from build123d import *

# Parameters (mm, degrees)
F0_R     = 88.9
F1_DEPTH = 50.8
F2_SIZE  = 25.4
F3_SIZE  = 25.39999
F4_R     = 30.4888877606
F5_DEPTH = 25.4
F6_R     = 25.39999
F7_W     = 8.3943400532
F7_H     = 6.7154671997
F7_W_2   = 8.0585591495
F7_W_3   = 7.0512406528
F7_H_2   = 7.0512406528
F7_H_3   = 7.722787559
F8_DEPTH = 12.7


# Not quite as in the source:
# - a fillet or chamfer is up to 0.001 mm smaller than in the source, because OpenCascade refuses the exact size


with BuildPart() as f1:
    # F0 (on Top) → F1 (new body)
    with BuildSketch(Plane.XY):
        Circle(F0_R)
    extrude(amount=F1_DEPTH)

    # F2
    f2_edges = [f1.edges().sort_by_distance(p)[0] for p in [
        (-88.9, 0, 50.8),
    ]]
    chamfer(f2_edges, length=F2_SIZE)

    # F3 (size 25.4 in the source; OpenCascade refuses exactly that, so slightly less here)
    f3_edges = [f1.edges().sort_by_distance(p)[0] for p in [
        (-88.9, 0, 0),
    ]]
    chamfer(f3_edges, length=F3_SIZE)

    # F4 (on face) → F5 (join)
    with BuildSketch(Plane.XY.offset(50.8)):
        Circle(F4_R)
    extrude(amount=F5_DEPTH)

    # F6 (radius 25.4 in the source; OpenCascade refuses exactly that, so slightly less here)
    f6_edges = [f1.edges().sort_by_distance(p)[0] for p in [
        (-30.488888, 0, 76.2),
    ]]
    fillet(f6_edges, radius=F6_R)

    # F7 (on face) → F8 (join)
    with BuildSketch(Plane(origin=(0, 0, 0), x_dir=(1, 0, 0), z_dir=(0, 0, -1))):
        with Locations((31.7305838689, 24.918817915)):
            Rectangle(F7_W, F7_H)
        with Locations((-29.8838298768, 24.918817915)):
            Rectangle(F7_W_2, F7_H)
        with Locations((-29.3801706284, -27.6297163218)):
            Rectangle(F7_W_3, F7_H_2)
        with Locations((31.7305838689, -27.2939428687)):
            Rectangle(F7_W, F7_H_3)
    extrude(amount=F8_DEPTH)


solid = f1.part
The model under review builds one solid part; all positions refer to its coordinate system, in mm. A direction names the side the tool comes from. Round coordinates to 2 decimals unless told otherwise and drop trailing zeros. Loops run counter-clockwise (first coordinate to the right, second up) from the corner with the lowest first, then second, coordinate; pieces in that order, holes last. Notation, with made-up numbers: (43.5, 65.5) -> (53.5, 65.5) arc R21 ccw to (53.5, 74.5) -> close; hole circle Ø11 at (39, 12). An arc over 180 degrees is marked (long way). One line per question, with ' | ' between items. Start each with the question number.
Item 1: For pin 1 (2 mm diameter, centred on y = -26.5, z = -4, fed in from -X); pin 2 (3 mm diameter, centred on y = -57.5, z = 40, fed in from +X); pin 3 (7.5 mm diameter, centred on y = -24.5, z = -6, fed in from +X), all flat-tipped, find the tip position at first contact; note any pin that passes through.
Item 2: Add section A-A, the plane z = 33.5. Write out the cut boundary in (x, y), then the cut area to 3 significant figures.
Item 3: Machinability: for faces 1 (the face through (32, -21.561, -6)), 2 (the face through (-30, -28.277, -6)), 3 (the face through (32, 31.155, -6)), 4 (the face through (27.533, 27, -6)), 5 (the face through (27, 15, 50.8)), which of the approach directions +Z, -Z, +X, -X, +Y, -Y give a long, thin tool a straight path to every point of the face, cutting with its end or side? Answer none if there is none.
Item 4: Add section B-B, the plane z = 9.5. Write out the cut boundary in (x, y), then the cut area to 3 significant figures.
Item 5: Wall thickness on line 1 along Z through (x, y) = (45.5, 10); line 2 along Y through (x, z) = (-10.5, 9); line 3 along X through (y, z) = (-17.5, 2): over which ranges is each line inside the solid? List them lowest first. Write a range as [from, to].
Item 6: Draft analysis for pull direction X (two halves, no side actions). For faces 6 (the face through (-33.913, -25, -6)), 7 (the face through (-25.855, -25, -6)), 8 (the face through (-29, 28, -12.7)), state which applies: +X half, -X half, draft (parallel to the pull), parting line (faces both ways), or undercut.
Return value:
1) pin 1: stops at x = -33.91 | pin 2: stops at x = 49.97 | pin 3: stops at x = 35.93
2) outline: circle Ø161.6 at (0, 0) | area: 20,500 mm2
3) face 1: -Z, +X, -X | face 2: -Z, +X, -X, -Y | face 3: -Z, +X, -X, +Y | face 4: -Z, +Y, -Y | face 5: +Z
4) outline: circle Ø146 at (0, 0) | area: 16,700 mm2
5) line 1: z = [0, 50.8] | line 2: y = [-71.74, 71.74] | line 3: x = [-63.12, 63.12]
6) face 6: -X half | face 7: undercut | face 8: draft
